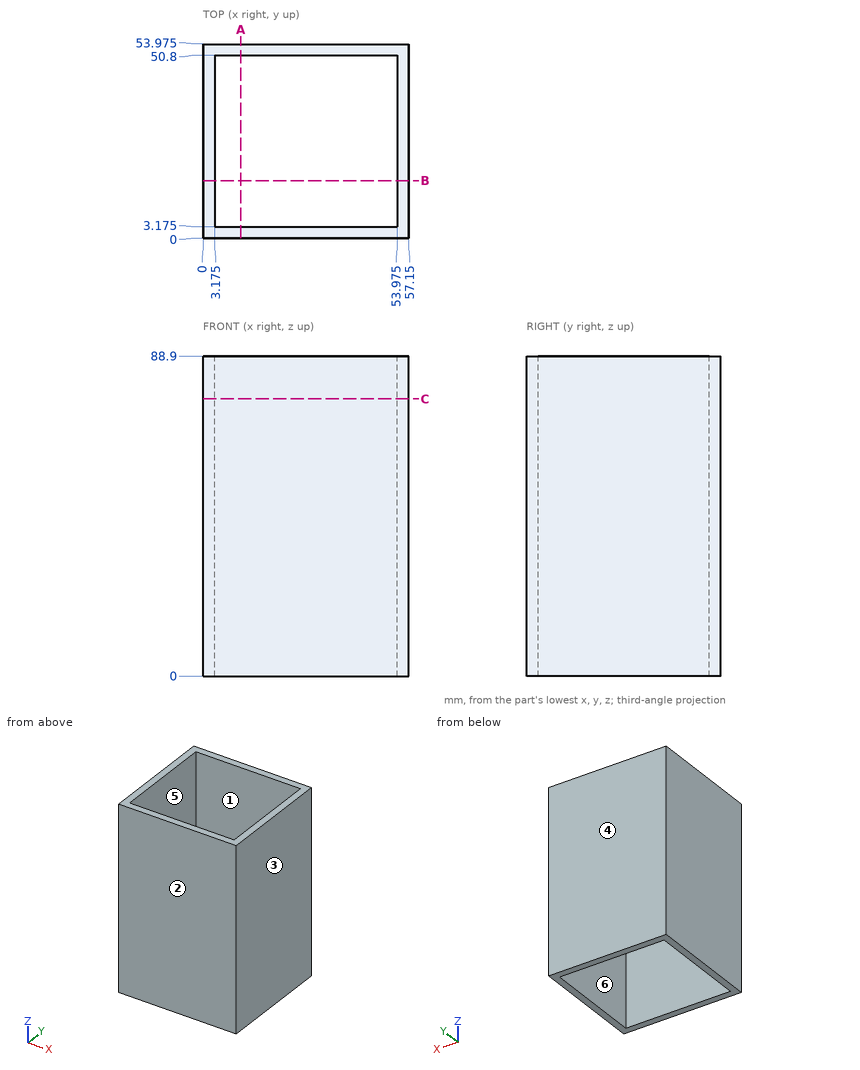
The figure shows three views and two pictorial views of one solid part (mm, origin at its lowest corner). Answer the questions. A direction names the side the tool comes from. Coordinates: 2 decimals unless noted, no trailing zeros. Loops run counter-clockwise (first coordinate to the right, second up) from the corner with the lowest first, then second, coordinate; pieces in that order, holes last. Notation, with made-up numbers: (25.5, 21.25) -> (57.5, 21.25) arc R17 cw to (57.5, 53.25) -> close; hole circle Ø7 at (45, -37). An arc over 180 degrees is marked (long way). Use one line per item in the form item = value. Start each with the question number.
Item 1: The part is cut by section B-B on y = 16. Determine the outline of the cut face in (x, z) (3 decimals).
Item 2: The mould has two halves that part along X. Classify the marked faces 3, 4, 5 and 6: released by +X, released by -X, zero draft, split by the parting line, or undercut.
Item 3: The part is cut by section C-C on z = 77. Determine the outline of the cut face in (x, y) (3 decimals), then the cut area to 3 significant figures.
Item 4: The part is cut by section A-A on x = 10.5. Determine the outline of the cut face in (y, z) (3 decimals).
Item 5: A flat-ended cylindrical pin translates along its axis: pin 1 Ø10 at (x, y) = (45, 32.5) entering from +Z. Find the tip coordinate at first contact, or state that the pin passes through.
Item 6: Consider L1, parallel to X at y = 10.5, z = 26.5 (3 decimals); L2, parallel to Y at x = 4.5, z = 23.5 (3 decimals). Determine where each line is inside the solid, lowest interval first. Write a range as [from, to].
Item 7: A tool of negligible diameter and unlimited length cuts with its end or side. For the marked faces 1 and 2, from which of +Z, -Z, +X, -X, +Y, -Y can it reach the whole face along a straight path? Write none if from no direction.
Answer key:
q1.outline = (0, 0) -> (3.175, 0) -> (3.175, 88.9) -> (0, 88.9) -> close; (53.975, 0) -> (57.15, 0) -> (57.15, 88.9) -> (53.975, 88.9) -> close
q2.face_3 = released by +X
q2.face_4 = zero draft
q2.face_5 = undercut
q2.face_6 = undercut
q3.outline = (0, 0) -> (57.15, 0) -> (57.15, 53.975) -> (0, 53.975) -> close; hole (3.175, 3.175) -> (53.975, 3.175) -> (53.975, 50.8) -> (3.175, 50.8) -> close
q3.area = 665 mm2
q4.outline = (0, 0) -> (3.175, 0) -> (3.175, 88.9) -> (0, 88.9) -> close; (50.8, 0) -> (53.975, 0) -> (53.975, 88.9) -> (50.8, 88.9) -> close
q5.pin_1 = through
q6.L1 = [0, 3.175], [53.975, 57.15]
q6.L2 = [0, 3.175], [50.8, 53.975]
q7.face_1 = +Z, -Z
q7.face_2 = +Z, -Z, +X, -X, -Y
